from build123d import *

# Parameters (mm, degrees)
SKETCH1_W           = 35
SKETCH1_H           = 35
BOSS_EXTRUDE1_DEPTH = 8
SKETCH2_W           = 5
SKETCH2_H           = 7
SKETCH2_W_2         = 7
SKETCH2_H_2         = 5
SKETCH2_R           = 1.5
CUT_EXTRUDE1_DEPTH  = 9
SKETCH2_5_R         = 4
SKETCH2_5_R_2       = 1.5
CUT_EXTRUDE2_DEPTH  = 4
SKETCH2_7_R         = 5
BOSS_EXTRUDE2_DEPTH = 98
SKETCH4_W           = 18
SKETCH4_H           = 18
BOSS_EXTRUDE3_DEPTH = 4
FILLET2_R           = 5


with BuildPart() as part:
    # Sketch1 → Boss-Extrude1 (new body)
    with BuildSketch(Plane(origin=(0, 0, 0), x_dir=(1, 0, 0), z_dir=(0, 1, 0))):
        with Locations((17.5, 17.5)):
            Rectangle(SKETCH1_W, SKETCH1_H)
    extrude(amount=BOSS_EXTRUDE1_DEPTH)

    # Sketch2 → Cut-Extrude1 (cut, through all)
    with BuildSketch(Plane.XZ):
        with Locations((32.5, -21.5)):
            Rectangle(SKETCH2_W, SKETCH2_H)
        with Locations((13.5, -32.5)):
            Rectangle(SKETCH2_W_2, SKETCH2_H_2)
        with Locations((2.5, -13.5)):
            Rectangle(SKETCH2_W, SKETCH2_H)
        with Locations((21.5, -2.5)):
            Rectangle(SKETCH2_W_2, SKETCH2_H_2)
        with Locations((11, -11)):
            Circle(SKETCH2_R)
        with Locations((24, -11)):
            Circle(SKETCH2_R)
        with Locations((11, -24)):
            Circle(SKETCH2_R)
        with Locations((24, -24)):
            Circle(SKETCH2_R)
    extrude(amount=-CUT_EXTRUDE1_DEPTH, mode=Mode.SUBTRACT)

    # Sketch2_5 → Cut-Extrude2 (cut)
    with BuildSketch(Plane.XZ):
        with Locations((6, -29)):
            Circle(SKETCH2_5_R)
        with Locations((29, -6)):
            Circle(SKETCH2_5_R)
        with Locations((11, -11)):
            Circle(SKETCH2_5_R_2)
    extrude(amount=-CUT_EXTRUDE2_DEPTH, mode=Mode.SUBTRACT)

    # Sketch2_7 → Boss-Extrude2 (add)
    with BuildSketch(Plane.XZ):
        with Locations((17.5, -17.5)):
            Circle(SKETCH2_7_R)
    extrude(amount=BOSS_EXTRUDE2_DEPTH)

    # Sketch4 → Boss-Extrude3 (add)
    with BuildSketch(Plane.XZ.offset(98)):
        with Locations((17.5, -17.5)):
            Rectangle(SKETCH4_W, SKETCH4_H)
    extrude(amount=BOSS_EXTRUDE3_DEPTH)

    # Fillet2
    fillet2_edges = [part.edges().sort_by_distance(p)[0] for p in [
        (0, 4, -35),
        (35, 4, -35),
        (35, 4, 0),
        (0, 4, 0),
    ]]
    fillet(fillet2_edges, radius=FILLET2_R)


solid = part.part
Verification items for the finished model (mm, model axes). A direction names the side the tool comes from. Give positions to 0.01 mm unless a question says otherwise; leave off trailing zeros. Write each loop counter-clockwise with the first axis right and the second up, starting at its lowest first coordinate (ties: lowest second). Pieces come first, ordered by that corner, then holes. Notation, with made-up numbers: M -8,74.5 L 3,74.5 A26 cw 3,100.5 Z; hole C -32.75,84 d4. An arc over 180 degrees is marked long. Write item = value, one per line.
(1) Sectioned sample at C-C (x = 29). Record the cut outline in (y, z), then the cut area to 3 significant figures.
Found:
outline = M 0,-35 L 8,-35 L 8,0 L 0,0 L 0,-2 L 4,-2 L 4,-10 L 0,-10 Z
area = 248 mm2
(2) Sectioned sample at D-D (y = -57). Record the cut outline in (x, z).
Found:
outline = C 17.5,-17.5 d10
(3) Go/stop test with flat-tipped pins: pin 1 Ø1.2 at (y, z) = (-101, -19.5) entering from -X; pin 2 Ø10 at (y, z) = (-65, -28.5) entering from +X; pin 3 Ø4 at (y, z) = (-43, -16.5) entering from -X; pin 4 Ø2.5 at (x, z) = (8, -29.5) entering from -Y. Record where each tip stops, or that it passes through.
Found:
pin_1 = 8.5
pin_2 = through
pin_3 = 12.5
pin_4 = 4
(4) Sectioned sample at B-B (z = -29). Record the cut outline in (x, y), then the cut area to 3 significant figures.
Found:
outline = M 0,0 L 2,0 L 2,4 L 10,4 L 10,0 L 35,0 L 35,8 L 0,8 Z
area = 248 mm2
(5) Sectioned sample at A-A (x = 11). Record the cut outline in (y, z), then the cut area to 3 significant figures.
Found:
outline = M -102,-26.5 L -98,-26.5 L -98,-8.5 L -102,-8.5 Z; M 0,-30 L 8,-30 L 8,-25.5 L 0,-25.5 Z; M 0,-22.5 L 8,-22.5 L 8,-12.5 L 0,-12.5 Z; M 0,-9.5 L 8,-9.5 L 8,0 L 0,0 Z
area = 264 mm2
(6) Access from +Z, -Z, +X, -X, +Y, -Y to the whole of each face (thin tool, end or side, straight path). Record for faces 1 (the face through (22.5, 3.94, -10.93)), 2 (the face through (18, 4, -3)), 3 (the face through (5, 4, -14)), 4 (the face through (17, 4, -33)), 5 (the face through (32, 4, -25)).
Found:
face_1 = +Y
face_2 = +Z, +Y, -Y
face_3 = -X, +Y, -Y
face_4 = -Z, +Y, -Y
face_5 = +X, +Y, -Y
(7) Material ranges on line 1 (Z direction, x = 24, y = 5); line 2 (Z direction, x = 11, y = 1); line 3 (Z direction, x = 29, y = 3), recorded low to high.
Found:
line_1 = -35 to -25.5, -22.5 to -12.5, -9.5 to -5
line_2 = -30 to -25.5, -22.5 to -12.5, -9.5 to 0
line_3 = -35 to -10, -2 to 0
